from build123d import *

# Parameters (mm, degrees)
SKETCH4_R           = 5.350481645
CUT_EXTRUDE2_DEPTH  = 3.683
FILLET1_R           = 1.27
SKETCH5_R           = 14.605
BOSS_EXTRUDE2_DEPTH = 101.6
BOSS_EXTRUDE3_START = 8.41019865
SKETCH6_R           = 14.605
SKETCH6_R_2         = 13.707723638
BOSS_EXTRUDE3_DEPTH = 8.41019865
DRAFT2_ANGLE        = -2
FILLET2_R           = 3.81
CUT_EXTRUDE3_DEPTH  = 7.366
DRAFT3_ANGLE        = 1


# Read off the part's stored shape, not the designer's step: Boss-Extrude1
with BuildPart() as part:
    # Sketch1 → Revolve1 (revolve)
    with BuildSketch(Plane.XY, mode=Mode.PRIVATE) as revolve1_sk:
        with BuildLine():
            Line((0, 0), (0, -7.747))
            Line((0, -7.747), (5.588, -7.747))
            ThreePointArc((5.588, -7.747), (11.354881185, -5.189962282), (13.707723638, 0.66319865))
            Line((13.707723638, 0.66319865), (13.145278313, 0.66319865))
            ThreePointArc((13.145278313, 0.66319865), (10.874067339, -4.877120177), (5.350481645, -7.188728508))
            Line((5.350481645, -7.188728508), (3.466052478, -3.180343574))
            Line((3.466052478, -3.180343574), (3.466052478, 0))
            Line((3.466052478, 0), (0, 0))
        make_face()
    revolve(revolve1_sk.sketch.rotate(Axis((0, 0, 0), (0, -1, 0)), 90), axis=Axis((0, 0, 0), (0, -1, 0)))

    # Boss-Extrude1 outline → Boss-Extrude1 (revolve)
    with BuildSketch(Plane.XY):
        with BuildLine():
            Line((13.707723638, -7.747), (13.707723638, 0.606068215))
            ThreePointArc((13.707723638, 0.606068215), (11.335005533, -5.21047892), (5.588, -7.747))
            Line((5.588, -7.747), (13.707723638, -7.747))
        make_face()
    revolve(axis=Axis((0, 0, 0), (0, 1, 0)))

    # Sketch4 → Cut-Extrude2 (cut)
    with BuildSketch(Plane(origin=(0, 0, 0), x_dir=(1, 0, 0), z_dir=(0, 1, 0))):
        Circle(SKETCH4_R)
    extrude(amount=-CUT_EXTRUDE2_DEPTH, mode=Mode.SUBTRACT)

    # Fillet1
    fillet1_edges = [part.edges().sort_by_distance(p)[0] for p in [
        (0, -7.188728508, -5.350481645),
    ]]
    fillet(fillet1_edges, radius=FILLET1_R)

    # Sketch5 → Boss-Extrude2 (add)
    with BuildSketch(Plane.XZ.offset(7.747)):
        with Locations(Location((0, 0, 0), (0, 0, 270))):
            Circle(SKETCH5_R)
    extrude(amount=BOSS_EXTRUDE2_DEPTH)

    # Sketch6 → Boss-Extrude3 (add)
    with BuildSketch(Plane(origin=(0, -7.747, 0), x_dir=(1, 0, 0), z_dir=(0, 1, 0)).offset(BOSS_EXTRUDE3_START)):
        with Locations(Location((0, 0, 0), (0, 0, 90))):
            Circle(SKETCH6_R)
        Circle(SKETCH6_R_2, mode=Mode.SUBTRACT)
    extrude(amount=-BOSS_EXTRUDE3_DEPTH)

    # Draft2
    draft2_faces = [part.faces().sort_by_distance(p)[0] for p in [
        (0, -54.341900675, 14.605),
    ]]
    draft(draft2_faces, Plane(origin=(13.707723638, 0.66319865, 0), x_dir=(0, 0, 1), z_dir=(0, 1, 0)), DRAFT2_ANGLE)

    # Fillet2
    fillet2_edges = [part.edges().sort_by_distance(p)[0] for p in [
        (0, -109.347, 10.763359211),
    ]]
    fillet(fillet2_edges, radius=FILLET2_R)

    # Sketch7 → Cut-Extrude3 (cut)
    with BuildSketch(Plane(origin=(0, -3.683, 0), x_dir=(1, 0, 0), z_dir=(0, 1, 0))):
        with BuildLine():
            Line((1.27, -1.4605), (-1.27, -1.4605))
            ThreePointArc((-1.27, -1.4605), (-1.9685, 0), (-1.27, 1.4605))
            Line((-1.27, 1.4605), (1.27, 1.4605))
            ThreePointArc((1.27, 1.4605), (1.9685, 0), (1.27, -1.4605))
        make_face()
    extrude(amount=-CUT_EXTRUDE3_DEPTH, mode=Mode.SUBTRACT)

    # Draft3
    draft3_faces = [part.faces().sort_by_distance(p)[0] for p in [
        (-1.9685, -7.366, 0),
        (0, -7.366, -1.4605),
        (0, -7.366, 1.4605),
        (1.9685, -7.366, 0),
    ]]
    draft(draft3_faces, Plane.ZX.offset(-3.683), DRAFT3_ANGLE)


solid = part.part
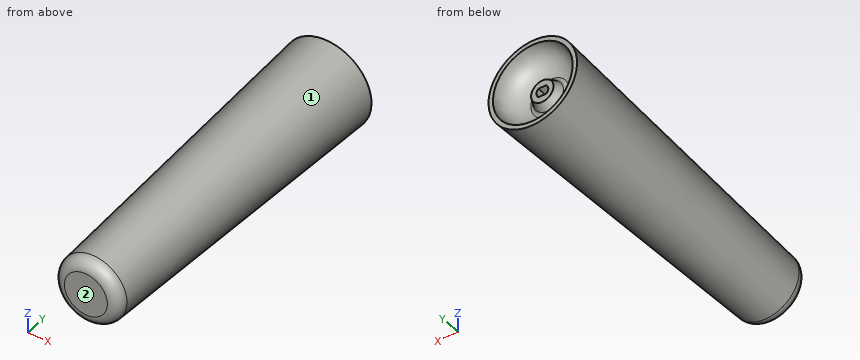
Build history of the part. All positions in model axes, mm. Face numbers are marked on the shaded views. A direction names the side the tool comes from. Round coordinates to 2 decimals unless told otherwise and drop trailing zeros. Loops run counter-clockwise (first coordinate to the right, second up) from the corner with the lowest first, then second, coordinate; pieces in that order, holes last. Notation, with made-up numbers: (26.25, -4) -> (47.25, -4) arc R20 ccw to (47.25, 0) -> close; hole circle Ø2 at (56.5, 6.5). An arc over 180 degrees is marked (long way). One line per item, written item: value. Start each with the question number.
Q1. 3-axis set-ups, long thin cutter, end or side, ignore diameter. For the marked faces 1 and 2: which of +Z, -Z, +X, -X, +Y, -Y reach the whole face in a straight line?
Q2. Cut at B-B on y = -15.5. List the corners of the cut face in (x, z).
Q3. Drop flat-ended pins along their axis: pin 1 Ø3.5 at (x, z) = (2, 0.5) entering from +Y; pin 2 Ø1.5 at (x, y) = (9.5, -47.5) entering from +Z; pin 3 Ø3 at (y, z) = (-12, 10) entering from -X; pin 4 Ø5 at (x, z) = (11, 2.5) entering from +Y. Give the stop position or say it passes through.
Q4. Cut at A-A on y = -89. List the corners of the cut face in (x, z), plus the area to 3 significant figures.
Q5. Probe line 1 along Z through (x, y) = (-6.25, -58); line 2 along Z through (x, y) = (0.25, -76); line 3 along X through (y, z) = (-82, 9). List the from-to ranges inside material, lowest first.
Computed:
1. face 1: -Y
1. face 2: +Z, -Z, +X, -X, -Y
2. outline: circle Ø28.08 at (0, 0)
3. pin 1: y = -3.68
3. pin 2: z = 9.51
3. pin 3: x = -11.33
3. pin 4: y = 0.66
4. outline: circle Ø22.95 at (0, 0)
4. area: 414 mm²
5. line 1: -10.89 to 10.89
5. line 2: -11.93 to 11.93
5. line 3: -7.5 to 7.5
